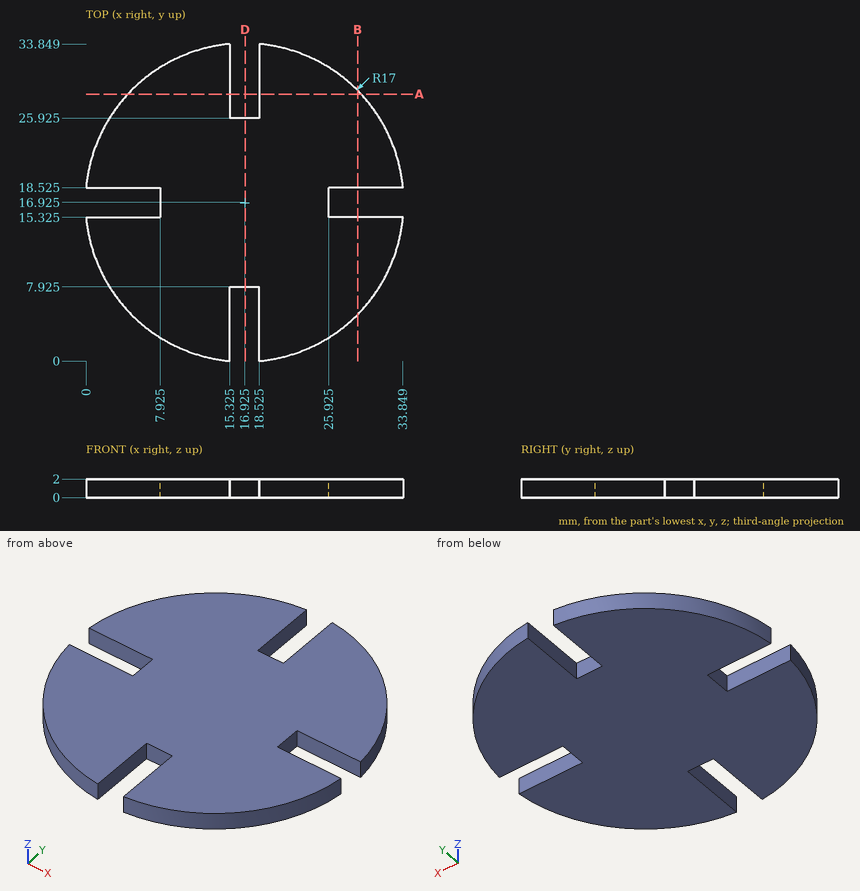
Design review of the part shown in the three views and the two pictorial views. Dimensions are in mm from the part's minimum x, y and z. Give positions to 0.01 mm unless a question says otherwise; leave off trailing zeros. Write each loop counter-clockwise with the first axis right and the second up, starting at its lowest first coordinate (ties: lowest second). Pieces come first, ordered by that corner, then holes. Notation, with made-up numbers: (-25.75, 39) - (10.25, 39) arc R23 cw to (10.25, 50) - close; hole circle Ø6 at (-14, -2). An arc over 180 degrees is marked (long way). Return JSON: item names as keys, results as strings. Group by question number.
(1) To check wall thickness, follow probe 1 along X at (y, z) = (2.5, 1.55) (1 decimal); probe 2 along Y at (x, z) = (28, 0.2) (1 decimal); probe 3 along X at (y, z) = (32, 0.6) (1 decimal). State the ranges of each line that lie inside material, in increasing order.
(2) We need section D-D, the plane x = 17. Give the boundary of the cut face in (y, z) (1 decimal).
(3) We need section B-B, the plane x = 29. Give the boundary of the cut face in (y, z) (1 decimal).
(4) We need section A-A, the plane y = 28.5. Give the boundary of the cut face in (x, z) (1 decimal).
(5) Insertion check: pin 1 (1 mm diameter, centred on y = 30.5, z = 1, fed in from -X); pin 2 (1 mm diameter, centred on x = 4, z = 1, fed in from +Y); pin 3 (1 mm diameter, centred on x = 17.5, z = 1, fed in from +Y) (1 decimal). Each pin has a flat end and moves straight along its axis. Give the tip position at first contact, or say it passes through.
Reported:
{
 "1": {"probe 1": "x = 7.9 to 15.3, 18.5 to 25.9", "probe 2": "y = 4 to 15.3, 18.5 to 29.8", "probe 3": "x = 9.1 to 15.3, 18.5 to 24.8"},
 "2": {"outline": "(7.9, 0) - (25.9, 0) - (25.9, 2) - (7.9, 2) - close"},
 "3": {"outline": "(5, 0) - (15.3, 0) - (15.3, 2) - (5, 2) - close; (18.5, 0) - (28.9, 0) - (28.9, 2) - (18.5, 2) - close"},
 "4": {"outline": "(4.5, 0) - (15.3, 0) - (15.3, 2) - (4.5, 2) - close; (18.5, 0) - (29.4, 0) - (29.4, 2) - (18.5, 2) - close"},
 "5": {"pin 1": "stops at x = 6.06", "pin 2": "stops at y = 28.53", "pin 3": "stops at y = 25.9"}
}
